Could you check a few things on this model? Use its own coordinates, in mm. Coordinates: 2 decimals unless noted, no trailing zeros. Write each loop counter-clockwise with the first axis right and the second up, starting at its lowest first coordinate (ties: lowest second). Pieces come first, ordered by that corner, then holes. Notation, with made-up numbers: M -9,-24.5 L 18,-24.5 A22 cw 18,9.5 Z; hole C 2.5,62.5 d5. An arc over 180 degrees is marked long. Write item = value, one per line.
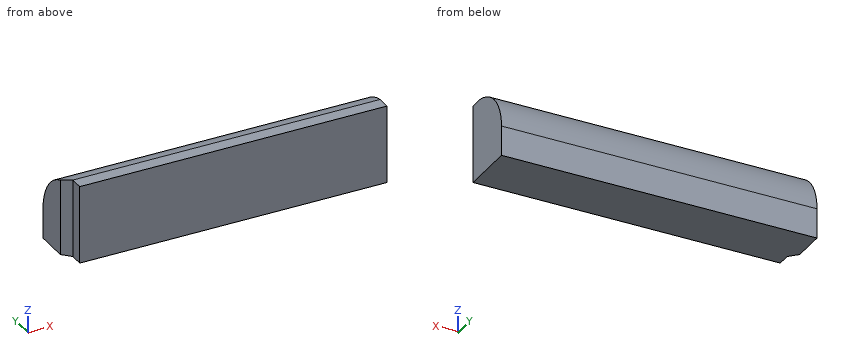
```python
from build123d import *

# Parameters (mm, degrees)
F0_W        = 194.6241557598
F0_H        = 48.2458211482
F1_DEPTH    = 25.4
F2_T1_DEPTH = 343.5218255279
F3_SIZE     = 5.08
F4_W        = 189.5441557598
F4_H        = 48.2458211482
F5_DEPTH    = 8.1318449229


# Not quite as in the source:
# - a fillet or chamfer that OpenCascade refuses, or shapes differently, is made with other operations: its cross-section is extruded or revolved along the edge and cut away or added


with BuildPart() as f1:
    # F0 (on Front) → F1 (new body)
    with BuildSketch(Plane.XZ):
        with Locations((-97.3120778799, 84.4252165407)):
            Rectangle(F0_W, F0_H)
    extrude(amount=F1_DEPTH)

    # F2: fillet of radius 30.1570992617 on 1 edges, made by hand

    # F2_s2 → F2_t1 (cut)
    with BuildSketch(Plane.YZ.offset(-269.0729906439)):
        with BuildLine():
            ThreePointArc((-25.4, 108.5481271148), (-7.2124816956, 98.3388553113), (0, 78.7685931612))
            Line((0, 78.7685931612), (0, 108.5481271148))
            Line((0, 108.5481271148), (-25.4, 108.5481271148))
        make_face()
    extrude(amount=F2_T1_DEPTH, mode=Mode.SUBTRACT)

    # F3
    f3_edges = [f1.edges().sort_by_distance(p)[0] for p in [
        (-194.624156, -25.4, 84.425217),
    ]]
    chamfer(f3_edges, length=F3_SIZE)

    # F4 (on face) → F5 (join)
    with BuildSketch(Plane.XZ.offset(25.4)):
        with Locations((-94.7720778799, 84.4252165407)):
            Rectangle(F4_W, F4_H)
    extrude(amount=F5_DEPTH)


solid = f1.part
```
Item 1: Imagine slicing it at B-B (y = -30). Write out the boundary of the cut face in (x, z), and give its area (3 significant figures).
Numbers:
outline = M -189.54,60.3 L 0,60.3 L 0,108.55 L -189.54,108.55 Z
area = 9,140 mm²
Item 2: I'm going to push flat-ended pins straight in: P1, Ø4, axis at y = -28.5, z = 73, coming from the -X side; P2, Ø3, axis at x = -27.5, y = -9, coming from the +Z side; P3, Ø3, axis at x = -42.5, y = -10.5, coming from the +Z side. Where does each tip first touch, or does it pass through?
Numbers:
P1 = -189.54
P2 = 101.64
P3 = 102.85
Item 3: Imagine slicing it at C-C (z = 103). Write out the boundary of the cut face in (x, y).
Numbers:
outline = M -194.62,-20.32 L -189.54,-25.4 L -189.54,-33.53 L 0,-33.53 L 0,-12.2 L -194.62,-12.2 Z
Item 4: Imagine slicing it at A-A (x = -176). Write out the boundary of the cut face in (y, z), and give its area (3 significant figures).
Numbers:
outline = M -33.53,60.3 L 0,60.3 L 0,78.77 A30.16 ccw -25.4,108.55 L -33.53,108.55 Z
area = 1,430 mm²
Item 5: If I drill on line 1 along X through (y, z) = (-27.5, 79); line 2 along Z through (x, y) = (-61, -10); line 3 along Y through (x, z) = (-126.5, 81), over which ranges is the centre line in solid material (lowest first)?
Numbers:
line_1 = -189.54 to 0
line_2 = 60.3 to 101.2
line_3 = -33.53 to -0.08
Item 6: Imagine slicing it at D-D (z = 84.5). Write out the boundary of the cut face in (x, y).
Numbers:
outline = M -194.62,-20.32 L -189.54,-25.4 L -189.54,-33.53 L 0,-33.53 L 0,-0.55 L -194.62,-0.55 Z
